Read the model definition and answer for the solid it produces. Units are mm, in the model's axes. Face numbers are marked on the shaded views. A direction names the side the tool comes from. Round coordinates to 2 decimals unless told otherwise and drop trailing zeros. Order: outer loops, then holes, each group sorted by start corner. A loop starts at its lowest first (then second) coordinate and runs counter-clockwise, first axis right, second up. Notation, with made-up numbers: (3, 89.5) - (11, 89.5) arc R28 ccw to (11, 128.5) - close; hole circle Ø5 at (-21.75, -4.75). An arc over 180 degrees is marked (long way). Put each result on its own line as item: value. Start each with the question number.
Q1. Find the intervals of material crossed by line 1 along Z through (x, y) = (-38, 11.5); line 2 along Y through (x, z) = (37, -6.5); line 3 along Y through (x, z) = (4, 44.5), in increasing order. Write a range as from..to.
Q2. Section A-A on y = -8.5 is taken. Give the vertices of the cut face in (x, z), then the cut area to 3 significant figures.
Q3. Which of the six approach directions +Z, -Z, +X, -X, +Y, -Y give full straight-line access (tool end or side, diameter ignored) to the marked faces 1, 2, 3, 4 and 5?
Q4. For a pull along Z with two mould halves and no side action, classify the marked faces 6, 7 and 8 as pulls with the +Z half, pulls with the -Z half, needs draft (parallel to the pull), parting line crosses it, or undercut.
Q5. Each of these flat-tipped pins is pushed along its axis until it touches: pin 1 Ø12 at (x, z) = (-26, -3) entering from -Y; pin 2 Ø6 at (x, y) = (-24.5, 10.5) entering from +Z; pin 3 Ø11 at (x, z) = (1.5, -38.5) entering from +Y; pin 4 Ø4.5 at (y, z) = (-8.5, 21) entering from +X. Where does it stop, or does it pass through?
Q6. Section D-D on y = 10.5 is taken. Give the vertices of the cut face in (x, z).
Q7. Section C-C on x = 30.5 is taken. Give the vertices of the cut face in (y, z), then the cut area to 3 significant figures.
from build123d import *

# Parameters (mm, degrees)
SKETCH1_W           = 100
SKETCH1_H           = 40
BOSS_EXTRUDE2_DEPTH = 16
SKETCH3_W           = 100
SKETCH3_H           = 30
CUT_EXTRUDE1_DEPTH  = 12
SKETCH4_W           = 10
SKETCH4_H           = 120
BOSS_EXTRUDE3_DEPTH = 5
SKETCH5_W           = 10
SKETCH5_H           = 5
BOSS_EXTRUDE4_DEPTH = 10
SKETCH6_W           = 10
SKETCH6_H           = 5
BOSS_EXTRUDE5_DEPTH = 10
FILLET1_R           = 5
FILLET2_R           = 5
FILLET3_R           = 5


with BuildPart() as part:
    # Sketch1 → Boss-Extrude2 (new body)
    with BuildSketch(Plane(origin=(0, 0, 0), x_dir=(1, 0, 0), z_dir=(0, 1, 0))):
        Rectangle(SKETCH1_W, SKETCH1_H)
    extrude(amount=BOSS_EXTRUDE2_DEPTH)

    # Sketch3 → Cut-Extrude1 (cut)
    with BuildSketch(Plane(origin=(0, 16, 0), x_dir=(1, 0, 0), z_dir=(0, 1, 0))):
        Rectangle(SKETCH3_W, SKETCH3_H)
    extrude(amount=-CUT_EXTRUDE1_DEPTH, mode=Mode.SUBTRACT)

    # Sketch4 → Boss-Extrude3 (add)
    with BuildSketch(Plane(origin=(0, 0, 0), x_dir=(-1, 0, 0), z_dir=(0, -1, 0))):
        Rectangle(SKETCH4_W, SKETCH4_H)
    extrude(amount=BOSS_EXTRUDE3_DEPTH)

    # Sketch5 → Boss-Extrude4 (add)
    with BuildSketch(Plane.XZ.offset(5)):
        with Locations((0, 57.5)):
            Rectangle(SKETCH5_W, SKETCH5_H)
    extrude(amount=BOSS_EXTRUDE4_DEPTH)

    # Sketch6 → Boss-Extrude5 (add)
    with BuildSketch(Plane.XZ.offset(5)):
        with Locations((0, -57.5)):
            Rectangle(SKETCH6_W, SKETCH6_H)
    extrude(amount=BOSS_EXTRUDE5_DEPTH)

    # Fillet1
    fillet1_edges = [part.edges().sort_by_distance(p)[0] for p in [
        (5, 0, 0),
    ]]
    fillet(fillet1_edges, radius=FILLET1_R - 0.0001)  # a hair under: the kernel refuses the full size

    # Fillet2
    fillet2_edges = [part.edges().sort_by_distance(p)[0] for p in [
        (-5, 0, 0),
    ]]
    fillet(fillet2_edges, radius=FILLET2_R - 0.0001)  # a hair under: the kernel refuses the full size

    # Fillet3
    fillet3_edges = [part.edges().sort_by_distance(p)[0] for p in [
        (0, 0, 20),
        (0, 0, -20),
        (-5, -2.49995, -20),
        (-5, -2.49995, 20),
        (5, -2.49995, 20),
        (5, -2.49995, -20),
    ]]
    fillet(fillet3_edges, radius=FILLET3_R - 0.0004)  # a hair under: the kernel refuses the full size


solid = part.part
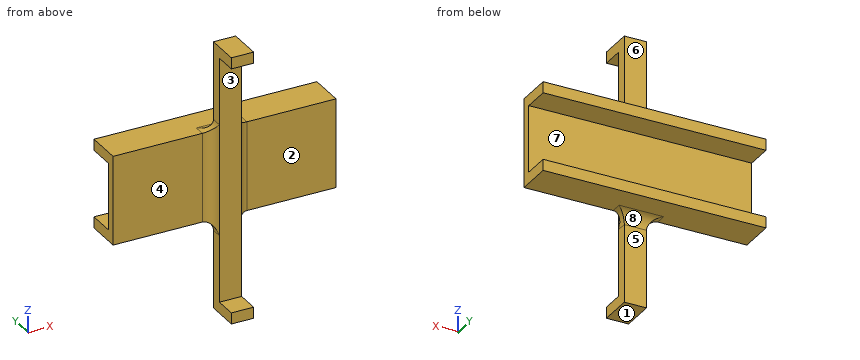
Findings:
1. line 1: -20..-15, 15..20
1. line 2: 0..4
1. line 3: -5..0
2. outline: (-5, -60) - (5, -60) - (5, -55) - (-5, -55) - close; (-5, 55) - (5, 55) - (5, 60) - (-5, 60) - close
2. area: 100 mm2
3. face 1: -Z, +X, -X, +Y, -Y
3. face 2: +Z, -Z, +X, -Y
3. face 3: +X, -X, -Y
3. face 4: +Z, -Z, -X, -Y
3. face 5: -Z, +X, -X, +Y
4. face 6: needs draft
4. face 7: undercut
4. face 8: pulls with the -Z half
5. pin 1: y = 0
5. pin 2: z = 20
5. pin 3: y = 0
5. pin 4: through
6. outline: (-50, -20) - (50, -20) - (50, -15) - (-50, -15) - close; (-50, 15) - (50, 15) - (50, 20) - (-50, 20) - close
7. outline: (0, -20) - (16, -20) - (16, -15) - (4, -15) - (4, 15) - (16, 15) - (16, 20) - (0, 20) - close
7. area: 280 mm2
